from build123d import *

# Parameters (mm, degrees)
SKETCH_W        = 169
SKETCH_H        = 16.5
SKETCH_W_2      = 131
SKETCH_H_2      = 150
PAD_DEPTH       = 79.5
SKETCH001_R     = 50
POCKET_DEPTH    = 79.501
POCKET001_DEPTH = 79.501
SKETCH003_W     = 30
SKETCH003_H     = 4
POCKET002_DEPTH = 79.501


with BuildPart() as part:
    # Sketch → Pad (new body)
    with BuildSketch(Plane.YZ):
        with Locations((84.5, 8.25)):
            Rectangle(SKETCH_W, SKETCH_H)
        with Locations((84.5, 91.5)):
            Rectangle(SKETCH_W_2, SKETCH_H_2)
    extrude(amount=PAD_DEPTH)

    # Sketch001 (on Face10 of Pad) → Pocket (cut, through all)
    with BuildSketch(Plane.YZ.offset(79.5)):
        with Locations((84.5, 60)):
            Circle(SKETCH001_R)
    extrude(amount=-POCKET_DEPTH, mode=Mode.SUBTRACT)

    # Sketch002 (on Face5 of Pocket) → Pocket001 (cut, through all)
    with BuildSketch(Plane.YZ.offset(79.5)):
        with BuildLine():
            Line((19, 83.870659), (32, 83.870659))
            ThreePointArc((137, 83.870652), (84.500002, 115.370656), (32, 83.870659))
            Line((150, 83.870652), (137, 83.870652))
            Line((183.643631, 183.574966), (150, 83.870652))
            Line((-15.737751, 179.863068), (183.643631, 183.574966))
            Line((19, 83.870659), (-15.737751, 179.863068))
        make_face()
    extrude(amount=-POCKET001_DEPTH, mode=Mode.SUBTRACT)

    # Sketch003 (on Face4 of Pocket001) → Pocket002 (cut, through all)
    with BuildSketch(Plane.YZ.offset(79.5)):
        with Locations((34, 60)):
            Rectangle(SKETCH003_W, SKETCH003_H)
    extrude(amount=-POCKET002_DEPTH, mode=Mode.SUBTRACT)


solid = part.part
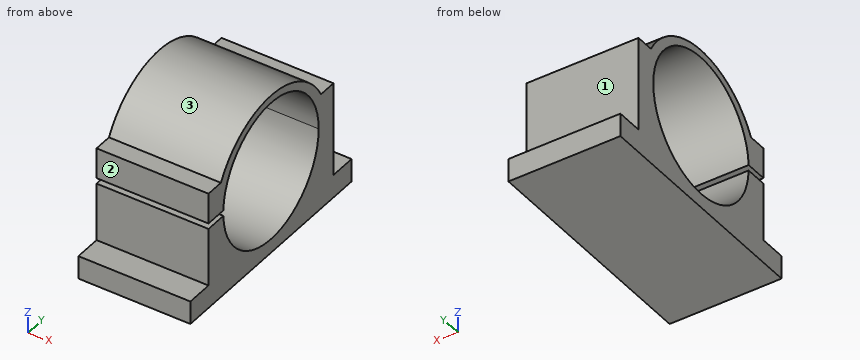
Could you check a few things on this model? Use its own coordinates, in mm. Face numbers are marked on the shaded views. A direction names the side the tool comes from. Coordinates: 2 decimals unless noted, no trailing zeros. Loops run counter-clockwise (first coordinate to the right, second up) from the corner with the lowest first, then second, coordinate; pieces in that order, holes last.
1. For the marked faces 1, 2 and 3, which set-ups out of +Z, -Z, +X, -X, +Y, -Y let a thin tool reach every point of the face, with its end or its side?
2. For P1, Ø4, axis at x = 49.5, y = 144, coming from the +Z side; P2, Ø9.5, axis at x = 44.5, y = 161, coming from the +Z side; P3, Ø3, axis at x = 61, z = 29, coming from the -Y side, each with a flat end and sliding along its axis, tell me the tip position at first contact or that it passes through.
3. I need wall thicknesses on L1, parallel to Z at x = 26.5, y = 85; L2, parallel to Z at x = 28.5, y = 27; L3, parallel to Z at x = 59.5, y = 139.5. Which ranges of each line are inside material? Lowest first, please.
4. Imagine slicing it at C-C (x = 55.5). Please give me the cut outline in (y, z), and give its area (3 significant figures).
5. Imagine slicing it at D-D (y = 144). Please give me the cut outline in (x, z), and give its area (3 significant figures).
6. Imagine slicing it at A-A (y = 24). Please give me the cut outline in (x, z).
7. Imagine slicing it at B-B (z = 26.5). Please give me the cut outline in (x, y), and give its area (3 significant figures).
Computed values:
1. face 1: +Z, +X, -X, +Y
1. face 2: +Z, +X, -X, -Y
1. face 3: +Z, +X, -X
2. P1: stops at z = 83.87
2. P2: stops at z = 16.5
2. P3: stops at y = 19
3. L1: z = 0 to 10, 110 to 115.37
3. L2: z = 0 to 58, 62 to 83.87
3. L3: z = 0 to 83.87
4. outline: (0, 0) - (169, 0) - (169, 16.5) - (150, 16.5) - (150, 83.87) - (137, 83.87) arc R59.5 ccw to (32, 83.87) - (19, 83.87) - (19, 62) - (34.54, 62) arc R50 cw (long way) to (34.54, 58) - (19, 58) - (19, 16.5) - (0, 16.5) - close
4. area: 6,050 mm2
5. outline: (0, 0) - (79.5, 0) - (79.5, 83.87) - (0, 83.87) - close
5. area: 6,670 mm2
6. outline: (0, 0) - (79.5, 0) - (79.5, 58) - (0, 58) - close; (0, 62) - (79.5, 62) - (79.5, 83.87) - (0, 83.87) - close
7. outline: (0, 19) - (79.5, 19) - (79.5, 47.38) - (0, 47.38) - close; (0, 121.62) - (79.5, 121.62) - (79.5, 150) - (0, 150) - close
7. area: 4,510 mm2
